The listing builds one solid part. Answer for the finished solid, in the listing's coordinates (mm). A direction names the side the tool comes from. Give positions to 0.01 mm unless a question says otherwise; leave off trailing zeros. Write each loop counter-clockwise with the first axis right and the second up, starting at its lowest first coordinate (ties: lowest second). Pieces come first, ordered by that corner, then holes. Notation, with made-up numbers: (17.25, 57) - (67.25, 57) arc R36 ccw to (67.25, 91) - close; hole circle Ø6 at (20.25, 85.25). An arc over 180 degrees is marked (long way). Answer in a Markdown table with one row per item. Add a question column.
from build123d import *

# Parameters (mm, degrees)
SKETCH016_W     = 5.5
SKETCH016_H     = 13.7
PAD006_DEPTH    = 4.6
POCKET007_DEPTH = 4
SKETCH018_W     = 13.7
SKETCH018_H     = 0.8
POCKET008_DEPTH = 1.8
SKETCH019_W     = 1.9
SKETCH019_H     = 0.9
POCKET009_DEPTH = 1


with BuildPart() as part:
    # Sketch016 → Pad006 (new body)
    with BuildSketch(Plane.XY):
        with Locations((-2.75, 0)):
            Rectangle(SKETCH016_W, SKETCH016_H)
    extrude(amount=PAD006_DEPTH)

    # Sketch017 → Pocket007 (cut)
    with BuildSketch(Plane.YZ):
        Polygon((-4, 4.6), (-4, 4.05), (-6.3, 4.05), (-6.3, 0.55), (6.3, 0.55), (6.3, 4.05), (4, 4.05), (4, 4.6), align=None)
    extrude(amount=-POCKET007_DEPTH, mode=Mode.SUBTRACT)

    # Sketch018 → Pocket008 (cut)
    with BuildSketch(Plane.YZ):
        with Locations((0, 2.9)):
            Rectangle(SKETCH018_W, SKETCH018_H)
    extrude(amount=-POCKET008_DEPTH, mode=Mode.SUBTRACT)

    # Sketch019 → Pocket009 (cut)
    with BuildSketch(Plane.XY.offset(4.6)):
        with Locations((-2.75, 5.75)):
            Rectangle(SKETCH019_W, SKETCH019_H)
        with Locations((-2.75, -5.75)):
            Rectangle(SKETCH019_W, SKETCH019_H)
    extrude(amount=-POCKET009_DEPTH, mode=Mode.SUBTRACT)


with BuildPart() as part_1:
    # Body008 placement: moved
    add(part.part.moved(Location((26, 0, -35.05))))


solid = part_1.part
1. Straight lines are drawn through the part: L1, parallel to Y at x = 23.9, z = -31.55; L2, parallel to Z at x = 25.3, y = 4.5; L3, parallel to Z at x = 23.95, y = 1.75. For each, find the intervals that lie inside material, in ascending order. Write a range as [from, to].
2. Section A-A (x = 24.4) is taken. Give the vertices of the cut face in (y, z), and give its area (3 significant figures).
3. Section D-D (z = -30.75) is taken. Give the vertices of the cut face in (x, y), and give its area (3 significant figures).
4. The mould has two halves that part along Z. Classify faces 3 (the face through (24, 6.3, -33)), 4 (the face through (26, 0, -34.8)), 5 (the face through (21, 0, -30.45)), 6 (the face through (24, 0, -34.5)): +Z half, -Z half, draft (parallel to the pull), parting line (faces both ways), or undercut.
5. Section B-B (y = -5.5) is taken. Give the vertices of the cut face in (x, z).
6. A tool of negligible diameter and unlimited length cuts with its end or side. For faces 1 (the face through (23, 6.85, -33)), 2 (the face through (24, -5, -31)), from which of +Z, -Z, +X, -X, +Y, -Y can it reach the whole face along a straight path? Write none if from no direction.
7. Section C-C (z = -32.25) is taken. Give the vertices of the cut face in (x, y).
Geometry check:
| question | item | result |
|---|---|---|
| 1 | L1 | [-6.85, -6.3], [6.3, 6.85] |
| 1 | L2 | [-35.05, -34.5], [-31, -30.45] |
| 1 | L3 | [-35.05, -34.5] |
| 2 | outline | (-6.85, -35.05) - (6.85, -35.05) - (6.85, -32.55) - (6.3, -32.55) - (6.3, -34.5) - (-6.3, -34.5) - (-6.3, -32.55) - (-6.85, -32.55) - close; (-6.85, -31.75) - (-6.3, -31.75) - (-6.3, -31) - (-4, -31) - (-4, -30.45) - (-6.85, -30.45) - close; (4, -31) - (6.3, -31) - (6.3, -31.75) - (6.85, -31.75) - (6.85, -30.45) - (4, -30.45) - close |
| 2 | area | 13.6 mm² |
| 3 | outline | (20.5, -6.85) - (26, -6.85) - (26, -4) - (22, -4) - (22, 4) - (26, 4) - (26, 6.85) - (20.5, 6.85) - close; hole (22.3, -6.2) - (24.2, -6.2) - (24.2, -5.3) - (22.3, -5.3) - close; hole (22.3, 5.3) - (24.2, 5.3) - (24.2, 6.2) - (22.3, 6.2) - close |
| 3 | area | 39.9 mm² |
| 4 | face 3 | undercut |
| 4 | face 4 | draft |
| 4 | face 5 | +Z half |
| 4 | face 6 | undercut |
| 5 | outline | (20.5, -35.05) - (26, -35.05) - (26, -34.5) - (22, -34.5) - (22, -31) - (22.3, -31) - (22.3, -30.45) - (20.5, -30.45) - close; (24.2, -31) - (26, -31) - (26, -30.45) - (24.2, -30.45) - close |
| 6 | face 1 | +Z, -Z, +X, -X, +Y |
| 6 | face 2 | +X |
| 7 | outline | (20.5, -6.85) - (24.2, -6.85) - (24.2, -6.3) - (22, -6.3) - (22, 6.3) - (24.2, 6.3) - (24.2, 6.85) - (20.5, 6.85) - close |
